```python
from build123d import *

# Parameters (mm, degrees)
F0_W     = 650
F0_H     = 700
F1_DEPTH = 30
F3_START = 350
F3_DEPTH = 50
F5_R     = 20
F6_W     = 1200
F6_H     = 600
F7_DEPTH = 1


with BuildPart() as f1:
    # F0 (on Top) → F1 (new body)
    with BuildSketch(Plane.XY):
        with Locations((325, 0)):
            Rectangle(F0_W, F0_H)
    extrude(amount=-F1_DEPTH)

    # F2 (on Right) → F3 (join)
    with BuildSketch(Plane.YZ.offset(F3_START)):
        Polygon((150, -30), (0, -30), (0, -650), (250, -650), (250, -630), (50, -600), align=None)
        Polygon((0, -650), (0, -30), (-150, -30), (-50, -600), (-250, -630), (-250, -650), align=None)
    extrude(amount=F3_DEPTH)

    # F4: F1 across plane


with BuildPart() as f1_1:
    add(f1.part)
    add(f1.part.mirror(Plane.YZ))

    # F5
    f5_edges = [f1_1.edges().sort_by_distance(p)[0] for p in [
        (0, 350, 0),
        (-650, 0, 0),
        (0, -350, 0),
        (650, 0, 0),
    ]]
    fillet(f5_edges, radius=F5_R)

    # F6 (on Top) → F7 (cut)
    with BuildSketch(Plane.XY):
        Rectangle(F6_W, F6_H)
    extrude(amount=-F7_DEPTH, mode=Mode.SUBTRACT)


solid = f1_1.part
```
Part model, mm, in its own coordinate system. A direction names the side the tool comes from. Give positions to 0.01 mm unless a question says otherwise; leave off trailing zeros. Order: outer loops, then holes, each group sorted by start corner. A loop starts at its lowest first (then second) coordinate and runs counter-clockwise, first axis right, second up. Notation, with made-up numbers: M -11,60.5 L 22,60.5 A13 cw 22,80.5 Z; hole C 43.25,77.5 d4. An arc over 180 degrees is marked long. Use a Markdown table: item, result. Add a question column.
(1) Drop flat-ended pins along their axis: P1, Ø12, axis at x = 35.5, y = -217.5, coming from the -Z side; P2, Ø10, axis at x = 447.5, y = 220.5, coming from the +Z side; P3, Ø6, axis at x = -382, z = -635.5, coming from the +Y side. Give the stop position or say it passes through.
(2) Saw through at A-A, the plane y = -194. Give the cut face in (x, z).
(3) Mould opens along Z. For faces 4 (the face through (350, -3, -336)), 5 (the face through (-374.65, 151.4, -615.21)), 6 (the face through (375, -3, -650)), 7 (the face through (-374.6, -100.7, -311)) say: +Z half, -Z half, draft (parallel to the pull), parting line (faces both ways), or undercut.
(4) Saw through at D-D, the plane y = 34. Give the cut face in (x, z).
(5) Saw through at C-C, the plane x = 493.5. Give the cut face in (y, z).
(6) 3-axis set-ups, long thin cutter, end or side, ignore diameter. For faces 1 (the face through (374.65, 151.4, -615.21)), 2 (the face through (-350, -3, -336)), 3 (the face through (-8, 4, -1)): which of +Z, -Z, +X, -X, +Y, -Y reach the whole face in a straight line?
(7) Probe line 1 along X through (y, z) = (55, -144.5); line 2 along Z through (x, y) = (21, -79); line 3 along Z through (x, y) = (394, -155). List the from-to ranges inside material, lowest first. Write a range as [from, to].
(8) Saw through at B-B, the plane z = -433. Give the cut face in (x, y).
Answer key:
| question | item | result |
|---|---|---|
| 1 | P1 | z = -30 |
| 1 | P2 | z = -1 |
| 1 | P3 | y = 250 |
| 2 | outline | M -650,-30 L 650,-30 L 650,-20 A20 ccw 630,0 L 600,0 L 600,-1 L -600,-1 L -600,0 L -630,0 A20 ccw -650,-20 Z; M -400,-650 L -350,-650 L -350,-621.6 L -400,-621.6 Z; M 350,-650 L 400,-650 L 400,-621.6 L 350,-621.6 Z |
| 3 | face 4 | draft |
| 3 | face 5 | undercut |
| 3 | face 6 | -Z half |
| 3 | face 7 | undercut |
| 4 | outline | M -650,-30 L -400,-30 L -400,-650 L -350,-650 L -350,-30 L 350,-30 L 350,-650 L 400,-650 L 400,-30 L 650,-30 L 650,-20 A20 ccw 630,0 L 600,0 L 600,-1 L -600,-1 L -600,0 L -630,0 A20 ccw -650,-20 Z |
| 5 | outline | M -350,-30 L 350,-30 L 350,-20 A20 ccw 330,0 L 300,0 L 300,-1 L -300,-1 L -300,0 L -330,0 A20 ccw -350,-20 Z |
| 6 | face 1 | +X, -X, +Y |
| 6 | face 2 | -Z, +Y, -Y |
| 6 | face 3 | +Z |
| 7 | line 1 | [-400, -350], [350, 400] |
| 7 | line 2 | [-30, -1] |
| 7 | line 3 | [-650, -615.75], [-30, -1] |
| 8 | outline | M -400,-79.3 L -350,-79.3 L -350,79.3 L -400,79.3 Z; M 350,-79.3 L 400,-79.3 L 400,79.3 L 350,79.3 Z |
